from build123d import *

# Parameters (mm, degrees)
M6X1_0_TAPPED_HOLE1_D           = 5
M6X1_0_TAPPED_HOLE1_DEPTH       = 45
M6X1_0_TAPPED_HOLE1_CSINK_D     = 6.05
M6X1_0_TAPPED_HOLE1_CSINK_ANGLE = 90
M6X1_0_TAPPED_HOLE1_TIP         = 1.502151548
SKETCH5_R                       = 3
CUT_EXTRUDE1_DEPTH              = 10
CUT_EXTRUDE1_DEPTH_BACK         = 10
CHAMFER1_SIZE                   = 1.5


with BuildPart() as part:
    # Sketch1 → Revolve4 (revolve)
    with BuildSketch(Plane(origin=(0, 0, 0), x_dir=(1, 0, 0), z_dir=(0, 1, 0))):
        Polygon((0, 6), (15, 6), (15, 9), (65, 9), (65, 6), (80, 6), (80, 0), (0, 0), align=None)
    revolve(axis=Axis((0, 0, 0), (1, 0, 0)))

    # M6x1.0 Tapped Hole1
    with Locations(Plane(origin=(80, 0, 0), x_dir=(0, 0, -1), z_dir=(1, 0, 0))):
        with Locations((0, 0)):
            CounterSinkHole(M6X1_0_TAPPED_HOLE1_D / 2, M6X1_0_TAPPED_HOLE1_CSINK_D / 2, depth=M6X1_0_TAPPED_HOLE1_DEPTH, counter_sink_angle=M6X1_0_TAPPED_HOLE1_CSINK_ANGLE)
            with Locations((0, 0, -(M6X1_0_TAPPED_HOLE1_DEPTH + M6X1_0_TAPPED_HOLE1_TIP / 2))):  # 118° drill point
                Cone(0, M6X1_0_TAPPED_HOLE1_D / 2, M6X1_0_TAPPED_HOLE1_TIP, mode=Mode.SUBTRACT)

    # Sketch5 → Cut-Extrude1 (cut, two sides)
    with BuildSketch(Plane.XY) as cut_extrude1_sk:
        with Locations((40, 0)):
            Circle(SKETCH5_R)
    extrude(amount=CUT_EXTRUDE1_DEPTH, mode=Mode.SUBTRACT)
    extrude(cut_extrude1_sk.sketch, amount=-CUT_EXTRUDE1_DEPTH_BACK, mode=Mode.SUBTRACT)

    # Chamfer1
    chamfer1_edges = [part.edges().sort_by_distance(p)[0] for p in [
        (0, 0, 6),
        (80, 0, 6),
    ]]
    chamfer(chamfer1_edges, length=CHAMFER1_SIZE)


solid = part.part
CAD build for the part. Positions are in the model's coordinates, mm. A direction names the side the tool comes from. Round coordinates to 2 decimals unless told otherwise and drop trailing zeros. Write each loop counter-clockwise with the first axis right and the second up, starting at its lowest first coordinate (ties: lowest second). Pieces come first, ordered by that corner, then holes.
(1) Slice it at B-B, the plane y = -1.25. Count the separate pieces of the cut face and the enclosed holes in it, and give its area (3 significant figures).
(2) Slice it at A-A, the plane x = 40. Write the cut outline in (y, z), and give its area (3 significant figures).
(3) Mould opens along X. For faces 1 (the face through (60.3, -2.44, -0.54)), 2 (the face through (15, -6, 2)), 3 (the face through (39.35, -2.93, 0.13)), 4 (the face through (65, -6, -2)) say: pulls with the +X half, pulls with the -X half, needs draft (parallel to the pull), parting line crosses it, or undercut.
(4) Drop flat-ended pins along their axis: P1, Ø1, axis at x = 32.5, z = -3, coming from the -Y side; P2, Ø1.5, axis at x = 43, y = -1.5, coming from the +Z side; P3, Ø3, axis at y = 0, z = 0, coming from the +X side. Give the stop position or say it passes through.
(5) Probe line 1 along Z through (x, y) = (36.3, 0); line 2 along X through (y, z) = (-4.5, 4.25); line 3 along Z through (x, y) = (48, 0.5). List the from-to ranges inside material, lowest first.
(6) Slice it at C-C, the plane z = 7. Write the cut outline in (x, y).
(7) 3-axis set-ups, long thin cutter, end or side, ignore diameter. For faces 5 (the face through (8, 0, 6)), 6 (the face through (0, 0, 0)), 7 (the face through (36.276, 0.751, 2.385)): which of +Z, -Z, +X, -X, +Y, -Y reach the whole face in a straight line?
(8) Slice it at D-D, the plane x = 10. Write the cut outline in (y, z), and give its area (3 significant figures).
From the geometry:
1. separate pieces: 3
1. enclosed holes: 0
1. area: 968 mm2
2. outline: (-3, -8.49) - (-3, 8.49) arc R9 ccw to start; (3, -8.49) arc R9 ccw to (3, 8.49) - close
2. area: 149 mm2
3. face 1: needs draft
3. face 2: pulls with the -X half
3. face 3: undercut
3. face 4: pulls with the +X half
4. P1: stops at y = -8.65
4. P2: stops at z = 8.97
4. P3: stops at x = 34.4
5. line 1: z = -9 to -2.5, 2.5 to 9
5. line 2: x = 15 to 65
5. line 3: z = -8.99 to -2.45, 2.45 to 8.99
6. outline: (15, -5.66) - (65, -5.66) - (65, 5.66) - (15, 5.66) - close; hole circle Ø6 at (40, 0)
7. face 5: -X
7. face 6: +Z, -Z, -X, +Y, -Y
7. face 7: +X
8. outline: circle Ø12 at (0, 0)
8. area: 113 mm2
